Can you work these out from the drawing? Everything is in mm from the part's minimum corner. A direction names the side the tool comes from. Coordinates: 2 decimals unless noted, no trailing zeros. Loops run counter-clockwise (first coordinate to the right, second up) from the corner with the lowest first, then second, coordinate; pieces in that order, holes last. Notation, with made-up numbers: M 84.5,-26.5 L 95.5,-26.5 A22 cw 95.5,-5.5 Z; hole C -24,-37 d8. An arc over 180 degrees is marked long. Write each question's results on one line, items separated by ' | '.
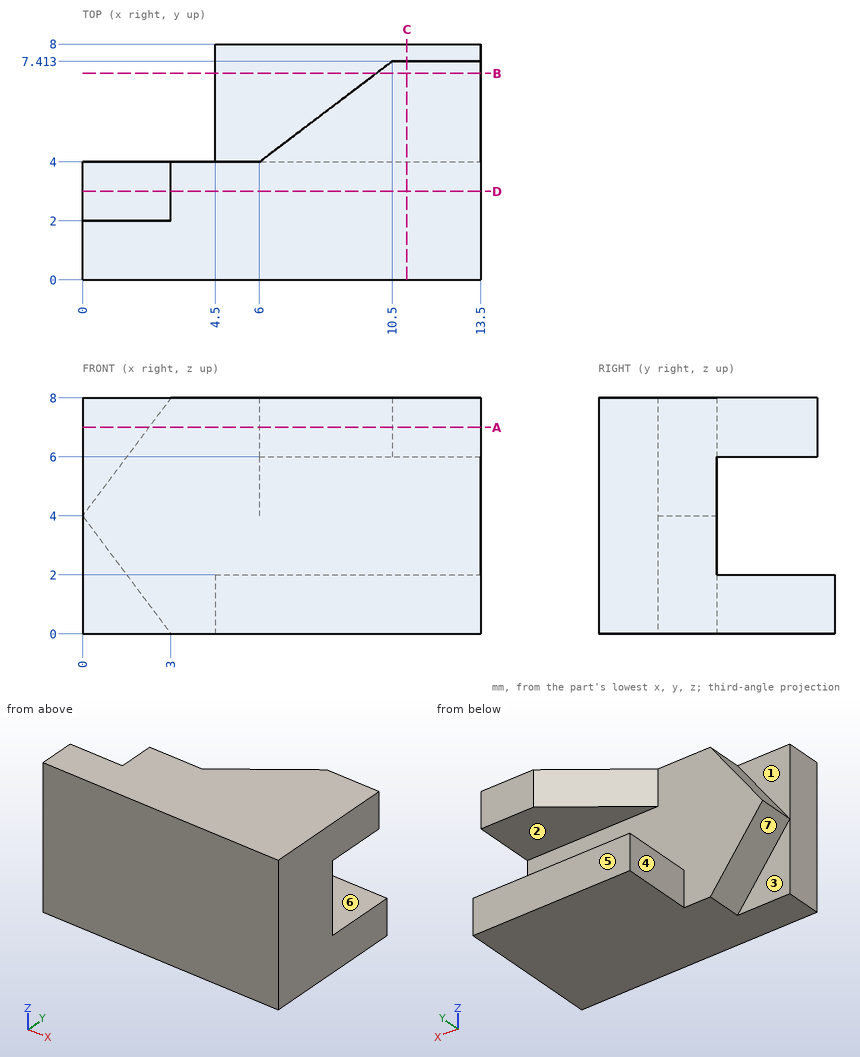
(1) If we mould it in two halves opening along Z, with no side actions, what happens to the marked faces 5, 6 and 7? For each: released by +Z, released by -Z, zero draft, split by the parting line, or undercut.
Reported:
face 5: zero draft | face 6: undercut | face 7: released by -Z
(2) Imagine slicing it at A-A, the plane z = 7. List the corners of the cut face in (x, y) for me.
Reported:
outline: M 0,0 L 13.5,0 L 13.5,7.41 L 10.5,7.41 L 6,4 L 2.25,4 L 2.25,2 L 0,2 Z
(3) Imagine slicing it at C-C, the plane x = 11. List the corners of the cut face in (y, z) for me.
Reported:
outline: M 0,0 L 8,0 L 8,2 L 4,2 L 4,6 L 7.41,6 L 7.41,8 L 0,8 Z
(4) Which directions (+Z, -Z, +X, -X, +Y, -Y) give clear straight access to the entire face, cutting with the end or side of a thin tool? Please do the marked faces 1, 2, 3 and 4.
Reported:
face 1: +Z, -X, +Y | face 2: +X, -X, +Y | face 3: -Z, -X, +Y | face 4: +Z, -Z, -X, +Y
(5) Imagine slicing it at B-B, the plane y = 7. List the corners of the cut face in (x, z) for me (1 decimal), and give its area (3 significant figures).
Reported:
outline: M 4.5,0 L 13.5,0 L 13.5,2 L 4.5,2 Z; M 10,6 L 13.5,6 L 13.5,8 L 10,8 Z | area: 25.1 mm2
(6) Imagine slicing it at D-D, the plane y = 3. List the corners of the cut face in (x, z) for me.
Reported:
outline: M 0,4 L 3,0 L 13.5,0 L 13.5,8 L 3,8 Z
(7) Will these pins go through, and if not, where does the flat tip stop? P1, Ø2, axis at x = 11.5, z = 6.5, coming from the +Y side; P2, Ø1.5, axis at x = 1.5, z = 6.5, coming from the +Y side; P3, Ø2.5, axis at x = 7.5, z = 5.5, coming from the +Y side.
Reported:
P1: stops at y = 7.41 | P2: stops at y = 4 | P3: stops at y = 6.01
(8) Please list where these lines run through material, in increasing order: probe 1 along Z at (x, y) = (9.25, 4.25); probe 2 along Z at (x, y) = (10, 7.25); probe 3 along Y at (x, z) = (5.75, 4). Write a range as from..to.
Reported:
probe 1: z = 0..2, 6..8 | probe 2: z = 0..2 | probe 3: y = 0..4
